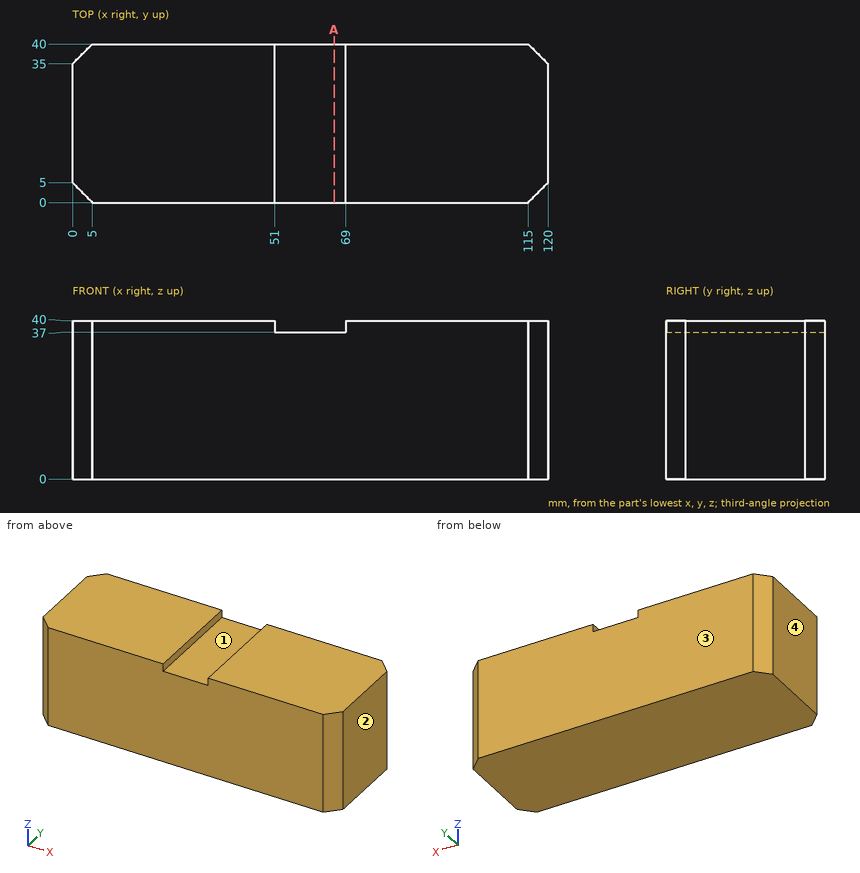
Job drawing, mm, ordinate dimensions from the low corner. One solid piece. Round coordinates to 2 decimals unless told otherwise and drop trailing zeros. Order: outer loops, then holes, each group sorted by start corner. A loop starts at its lowest first (then second) coordinate and runs counter-clockwise, first axis right, second up. Notation, with made-up numbers: (-32.75, 5) -> (-6.75, 5) arc R22 ccw to (-6.75, 31) -> close; hole circle Ø9 at (65, 36). An arc over 180 degrees is marked (long way). Answer in a Markdown table with one row per item.
1) Band-saw the part on A-A on x = 66. Give the cut face in (y, z).
Values:
| item | result |
|---|---|
| outline | (0, 0) -> (40, 0) -> (40, 37) -> (0, 37) -> close |
2) Wall check: L1, parallel to X at y = 4, z = 4.5; L2, parallel to X at y = 4.5, z = 25. Give the ranges that are in metal, low to high.
Values:
| item | result |
|---|---|
| L1 | 1 to 119 |
| L2 | 0.5 to 119.5 |
3) Mould opens along X. For the marked faces 1, 2, 3 and 4 say: released by +X, released by -X, zero draft, split by the parting line, or undercut.
Values:
| item | result |
|---|---|
| face 1 | undercut |
| face 2 | released by +X |
| face 3 | zero draft |
| face 4 | released by -X |
